Input: part model. Units: mm. Frame: model coordinates. Coordinates: 2 decimals unless noted, no trailing zeros. Write each loop counter-clockwise with the first axis right and the second up, starting at its lowest first coordinate (ties: lowest second). Pieces come first, ordered by that corner, then holes. Notation, with made-up numbers: (79.5, 39) -> (93.5, 39) arc R24 ccw to (93.5, 53) -> close; hole circle Ø2 at (45, -6.75). An arc over 180 degrees is marked (long way). Use one line per item in the form item = value. Start each with the question number.
(1) Cut plane A-A on x = 0. Return the cut outline in (y, z) (3 decimals).
(2) First-contact query: pin 1 (1.5 mm diameter, centred on y = -3.5, z = 3, fed in from -X) (3 decimals); pin 2 (3 mm diameter, centred on x = -18, z = 1, fed in from -Y); pin 3 (2 mm diameter, centred on y = -5, z = 1.5, fed in from -X). Flat tips, straight axial feed; report the tip coordinate or a pass-through.
(3) Ray query, line 1 along Y through (x, z) = (0, 1.15) (3 decimals); line 2 along X through (y, z) = (1.75, 3.9); line 3 along Y through (x, z) = (-15.15, 2.3) (3 decimals). Return the intervals inside material, ascending.
(4) Cut plane B-B on y = 6. State how many separate pieces and enclosed holes the cut face has, plus the area to 3 significant figures.
(5) Pull-direction query (X, two-part tool) for faces 1 (the face through (-21.72, 0.29, 2.46)), 2 (the face through (-0.093, -10.856, 2.479)), 3 (the face through (-10.89, -8.32, 2.48)), 4 (the face through (2, -7, 5)); classes: released by +X, released by -X, zero draft, split by the parting line, or undercut.
```python
from build123d import *

# Parameters (mm, degrees)
F0_R     = 6.575
F1_DEPTH = 5
F2_R     = 1


with BuildPart() as f1:
    # F0 (on Top) → F1 (new body)
    with BuildSketch(Plane.XY):
        with BuildLine():
            ThreePointArc((-6.389604, 8.776923), (-10.769802, 8.318304), (-15.15, 8.776923))
            ThreePointArc((-15.15, 8.776923), (-23.926923, 0), (-15.15, -8.776923))
            ThreePointArc((-15.15, -8.776923), (-10.769802, -8.318304), (-6.389604, -8.776923))
            ThreePointArc((-6.389604, -8.776923), (0, -10.856399), (6.389604, -8.776923))
            ThreePointArc((6.389604, -8.776923), (10.769802, -8.318304), (15.15, -8.776923))
            ThreePointArc((15.15, -8.776923), (23.926923, 0), (15.15, 8.776923))
            ThreePointArc((15.15, 8.776923), (10.769802, 8.318304), (6.389604, 8.776923))
            ThreePointArc((6.389604, 8.776923), (0, 10.856399), (-6.389604, 8.776923))
        make_face()
        with Locations((-15.15, 0)):
            Circle(F0_R, mode=Mode.SUBTRACT)
        Circle(F0_R, mode=Mode.SUBTRACT)
        with BuildLine():
            ThreePointArc((21.725, 0), (15.15, -6.575), (8.575, 0))
            ThreePointArc((8.575, 0), (15.15, 6.575), (21.725, 0))
        make_face(mode=Mode.SUBTRACT)
    extrude(amount=F1_DEPTH)

    # F2
    f2_edges = [f1.edges().sort_by_distance(p)[0] for p in [
        (-15.15, 8.776923, 2.5),
        (-15.15, -8.776923, 2.5),
        (-23.926923, 0, 0),
        (-23.926923, 0, 5),
        (-6.389604, -8.776923, 2.5),
        (-10.769802, -8.318304, 0),
        (-10.769802, -8.318304, 5),
        (6.389604, -8.776923, 2.5),
        (0, -10.856399, 0),
        (0, -10.856399, 5),
        (15.15, -8.776923, 2.5),
        (10.769802, -8.318304, 0),
        (10.769802, -8.318304, 5),
        (15.15, 8.776923, 2.5),
        (23.926923, 0, 0),
        (23.926923, 0, 5),
        (6.389604, 8.776923, 2.5),
        (10.769802, 8.318304, 0),
        (10.769802, 8.318304, 5),
        (-6.389604, 8.776923, 2.5),
        (0, 10.856399, 0),
        (0, 10.856399, 5),
        (-10.769802, 8.318304, 0),
        (-10.769802, 8.318304, 5),
    ]]
    fillet(f2_edges, radius=F2_R)


solid = f1.part
```
Values:
q1.outline = (-10.856, 1) arc R1 ccw to (-9.856, 0) -> (-6.575, 0) -> (-6.575, 5) -> (-9.856, 5) arc R1 ccw to (-10.856, 4) -> close; (6.575, 0) -> (9.856, 0) arc R1 ccw to (10.856, 1) -> (10.856, 4) arc R1 ccw to (9.856, 5) -> (6.575, 5) -> close
q2.pin_1 = -23.485
q2.pin_2 = -8.67
q2.pin_3 = -22.96
q3.line_1 = -10.856 to -6.575, 6.575 to 10.856
q3.line_2 = -23.75 to -21.49, -8.81 to -6.34, 6.34 to 8.81, 21.49 to 23.75
q3.line_3 = -8.771 to -6.575, 6.575 to 8.771
q4.separate_pieces = 4
q4.enclosed_holes = 0
q4.area = 134 mm2
q5.face_1 = undercut
q5.face_2 = split by the parting line
q5.face_3 = undercut
q5.face_4 = zero draft
